from build123d import *

# Parameters (mm, degrees)
F1_DEPTH = 6.35


# Not quite as in the source:
# - a length typed as a fraction of an inch, garbled in the dataset ("3 / 203.2 mm" for 3/8 in), is restored


with BuildPart() as f1:
    # F0 (on Front) → F1 (new body)
    with BuildSketch(Plane.XZ):
        with BuildLine():
            ThreePointArc((24.579061552, 28.3529026657), (9.5195561517, 35.7531570559), (-5.2125295141, 27.720839839))
            ThreePointArc((-5.2125295141, 27.720839839), (-29.7447728029, 24.816757347), (-32.6261176355, 0.281833099))
            ThreePointArc((-32.6261176355, 0.281833099), (-47.6586884842, -25.465181848), (-20.6299769397, -38.0483339671))
            ThreePointArc((-20.6299769397, -38.0483339671), (-9.7842016961, -50.4339494071), (5.705863164, -44.8579112888))
            ThreePointArc((5.705863164, -44.8579112888), (16.7493256027, -47.8238039479), (27.779373908, -44.8084074092))
            ThreePointArc((27.779373908, -44.8084074092), (48.6340616912, -53.8941801606), (64.9161967707, -38.0082950333))
            ThreePointArc((64.9161967707, -38.0082950333), (88.8664062791, -22.618688114), (76.0994801139, 2.8265105082))
            ThreePointArc((76.0994801139, 2.8265105082), (70.0975710942, 28.7139027136), (43.5306278663, 28.0994805429))
            ThreePointArc((43.5306278663, 28.0994805429), (34.0869435906, 30.6266295541), (24.579061552, 28.3529026657))
        make_face()
        with BuildLine():
            ThreePointArc((9.9552140403, -22.4611988481), (10.8253405255, -21.564938524), (11.9872140403, -21.1061873886))
            Line((11.9872140403, -21.1061873886), (12.5920123004, -14.8077944269))
            Line((12.5920123004, -14.8077944269), (12.0265549094, -13.8484140251))
            Line((12.0265549094, -13.8484140251), (13.1350774738, -13.9548590377))
            Line((13.1350774738, -13.9548590377), (13.5390697269, -12.9171003587))
            Line((13.5390697269, -12.9171003587), (13.7382008585, -14.0127734892))
            Line((13.7382008585, -14.0127734892), (14.8467234229, -14.1192185018))
            Line((14.8467234229, -14.1192185018), (14.1090343836, -14.9534652864))
            Line((14.1090343836, -14.9534652864), (13.5042361235, -21.2518582481))
            ThreePointArc((13.5042361235, -21.2518582481), (14.3943138922, -21.7735734557), (15.0519583946, -22.5685130135))
            Line((15.0519583946, -22.5685130135), (21.1719606568, -20.9619305704))
            Line((21.1719606568, -20.9619305704), (21.788173451, -20.0343344251))
            Line((21.788173451, -20.0343344251), (22.0579849941, -21.114776255))
            Line((22.0579849941, -21.114776255), (23.1710785379, -21.1490629746))
            Line((23.1710785379, -21.1490629746), (22.2940630935, -21.8353549873))
            Line((22.2940630935, -21.8353549873), (22.5638746366, -22.9157968171))
            Line((22.5638746366, -22.9157968171), (21.5589198477, -22.4359857202))
            Line((21.5589198477, -22.4359857202), (15.4389175856, -24.0425681633))
            ThreePointArc((15.4389175856, -24.0425681633), (15.2565271687, -25.0580281222), (14.7374718125, -25.9496596209))
            Line((14.7374718125, -25.9496596209), (18.3579193376, -31.1388690552))
            Line((18.3579193376, -31.1388690552), (19.4102498473, -31.5032188374))
            Line((19.4102498473, -31.5032188374), (18.4969454746, -32.1404200522))
            Line((18.4969454746, -32.1404200522), (18.8616543221, -33.1926261736))
            Line((18.8616543221, -33.1926261736), (18.0000377843, -32.487099982))
            Line((18.0000377843, -32.487099982), (17.0867334116, -33.1243011968))
            Line((17.0867334116, -33.1243011968), (17.1080536411, -32.0108849615))
            Line((17.1080536411, -32.0108849615), (13.487606116, -26.8216755271))
            ThreePointArc((13.487606116, -26.8216755271), (12.471606116, -27.0010332485), (11.455606116, -26.8216755271))
            Line((11.455606116, -26.8216755271), (7.835158591, -32.0108849615))
            Line((7.835158591, -32.0108849615), (7.8564698266, -33.124301369))
            Line((7.8564698266, -33.124301369), (6.9431654539, -32.4871001542))
            Line((6.9431654539, -32.4871001542), (6.0815366025, -33.1926113076))
            Line((6.0815366025, -33.1926113076), (6.4462638144, -32.1404115518))
            Line((6.4462638144, -32.1404115518), (5.5329594417, -31.5032103369))
            Line((5.5329594417, -31.5032103369), (6.5852928945, -31.1388690552))
            Line((6.5852928945, -31.1388690552), (10.2057404195, -25.9496596209))
            ThreePointArc((10.2057404195, -25.9496596209), (9.6657394654, -24.9991764128), (9.5065515642, -23.9176596209))
            Line((9.5065515642, -23.9176596209), (3.4595978764, -22.0548966372))
            Line((3.4595978764, -22.0548966372), (2.4058730089, -22.4152268431))
            Line((2.4058730089, -22.4152268431), (2.7337236859, -21.3509487369))
            Line((2.7337236859, -21.3509487369), (1.7987755438, -20.7459314434))
            Line((1.7987755438, -20.7459314434), (2.9121035894, -20.7719048279))
            Line((2.9121035894, -20.7719048279), (3.2399542664, -19.7076267216))
            Line((3.2399542664, -19.7076267216), (3.9082603526, -20.5984358645))
            Line((3.9082603526, -20.5984358645), (9.9552140403, -22.4611988481))
        make_face(mode=Mode.SUBTRACT)
        with BuildLine():
            ThreePointArc((-14.9548382666, 14.9038782153), (-14.0847117815, 15.8001385395), (-12.9228382666, 16.2588896749))
            Line((-12.9228382666, 16.2588896749), (-12.3180400065, 22.5572826366))
            Line((-12.3180400065, 22.5572826366), (-12.8834973975, 23.5166630384))
            Line((-12.8834973975, 23.5166630384), (-11.7749748332, 23.4102180258))
            Line((-11.7749748332, 23.4102180258), (-11.37098258, 24.4479767047))
            Line((-11.37098258, 24.4479767047), (-11.1718514484, 23.3523035743))
            Line((-11.1718514484, 23.3523035743), (-10.0633288841, 23.2458585617))
            Line((-10.0633288841, 23.2458585617), (-10.8010179234, 22.411611777))
            Line((-10.8010179234, 22.411611777), (-11.4058161835, 16.1132188153))
            ThreePointArc((-11.4058161835, 16.1132188153), (-10.5157384147, 15.5915036078), (-9.8580939123, 14.7965640499))
            Line((-9.8580939123, 14.7965640499), (-3.7380916502, 16.4031464931))
            Line((-3.7380916502, 16.4031464931), (-3.121878856, 17.3307426383))
            Line((-3.121878856, 17.3307426383), (-2.8520673129, 16.2503008085))
            Line((-2.8520673129, 16.2503008085), (-1.7389737691, 16.2160140888))
            Line((-1.7389737691, 16.2160140888), (-2.6159892135, 15.5297220761))
            Line((-2.6159892135, 15.5297220761), (-2.3461776704, 14.4492802463))
            Line((-2.3461776704, 14.4492802463), (-3.3511324592, 14.9290913433))
            Line((-3.3511324592, 14.9290913433), (-9.4711347214, 13.3225089001))
            ThreePointArc((-9.4711347214, 13.3225089001), (-9.6535251382, 12.3070489413), (-10.1725804944, 11.4154174426))
            Line((-10.1725804944, 11.4154174426), (-6.5521329694, 6.2262080082))
            Line((-6.5521329694, 6.2262080082), (-5.4998024597, 5.8618582261))
            Line((-5.4998024597, 5.8618582261), (-6.4131068324, 5.2246570112))
            Line((-6.4131068324, 5.2246570112), (-6.0483979848, 4.1724508898))
            Line((-6.0483979848, 4.1724508898), (-6.9100145227, 4.8779770815))
            Line((-6.9100145227, 4.8779770815), (-7.8233188953, 4.2407758666))
            Line((-7.8233188953, 4.2407758666), (-7.8019986659, 5.354192102))
            Line((-7.8019986659, 5.354192102), (-11.4224461909, 10.5434015363))
            ThreePointArc((-11.4224461909, 10.5434015363), (-12.4384461909, 10.3640438149), (-13.4544461909, 10.5434015363))
            Line((-13.4544461909, 10.5434015363), (-17.0748937159, 5.354192102))
            Line((-17.0748937159, 5.354192102), (-17.0535824803, 4.2407756944))
            Line((-17.0535824803, 4.2407756944), (-17.966886853, 4.8779769093))
            Line((-17.966886853, 4.8779769093), (-18.8285157045, 4.1724657558))
            Line((-18.8285157045, 4.1724657558), (-18.4637884925, 5.2246655117))
            Line((-18.4637884925, 5.2246655117), (-19.3770928652, 5.8618667265))
            Line((-19.3770928652, 5.8618667265), (-18.3247594124, 6.2262080082))
            Line((-18.3247594124, 6.2262080082), (-14.7043118874, 11.4154174426))
            ThreePointArc((-14.7043118874, 11.4154174426), (-15.2443128415, 12.3659006506), (-15.4035007427, 13.4474174426))
            Line((-15.4035007427, 13.4474174426), (-21.4504544305, 15.3101804262))
            Line((-21.4504544305, 15.3101804262), (-22.5041792981, 14.9498502204))
            Line((-22.5041792981, 14.9498502204), (-22.176328621, 16.0141283266))
            Line((-22.176328621, 16.0141283266), (-23.1112767632, 16.61914562))
            Line((-23.1112767632, 16.61914562), (-21.9979487176, 16.5931722356))
            Line((-21.9979487176, 16.5931722356), (-21.6700980405, 17.6574503418))
            Line((-21.6700980405, 17.6574503418), (-21.0017919544, 16.7666411989))
            Line((-21.0017919544, 16.7666411989), (-14.9548382666, 14.9038782153))
        make_face(mode=Mode.SUBTRACT)
        with BuildLine():
            ThreePointArc((48.6740988512, 2.4488521783), (49.5442253363, 3.3451125024), (50.7060988512, 3.8038636378))
            Line((50.7060988512, 3.8038636378), (51.3108971112, 10.1022565995))
            Line((51.3108971112, 10.1022565995), (50.7454397202, 11.0616370013))
            Line((50.7454397202, 11.0616370013), (51.8539622846, 10.9551919887))
            Line((51.8539622846, 10.9551919887), (52.2579545378, 11.9929506677))
            Line((52.2579545378, 11.9929506677), (52.4570856693, 10.8972775372))
            Line((52.4570856693, 10.8972775372), (53.5656082337, 10.7908325246))
            Line((53.5656082337, 10.7908325246), (52.8279191944, 9.95658574))
            Line((52.8279191944, 9.95658574), (52.2231209343, 3.6581927783))
            ThreePointArc((52.2231209343, 3.6581927783), (53.113198703, 3.1364775707), (53.7708432054, 2.3415380128))
            Line((53.7708432054, 2.3415380128), (59.8908454676, 3.948120456))
            Line((59.8908454676, 3.948120456), (60.5070582618, 4.8757166012))
            Line((60.5070582618, 4.8757166012), (60.7768698049, 3.7952747714))
            Line((60.7768698049, 3.7952747714), (61.8899633487, 3.7609880518))
            Line((61.8899633487, 3.7609880518), (61.0129479043, 3.0746960391))
            Line((61.0129479043, 3.0746960391), (61.2827594474, 1.9942542093))
            Line((61.2827594474, 1.9942542093), (60.2778046585, 2.4740653062))
            Line((60.2778046585, 2.4740653062), (54.1578023964, 0.8674828631))
            ThreePointArc((54.1578023964, 0.8674828631), (53.9754119795, -0.1479770958), (53.4563566233, -1.0396085945))
            Line((53.4563566233, -1.0396085945), (57.0768041484, -6.2288180289))
            Line((57.0768041484, -6.2288180289), (58.1291346581, -6.593167811))
            Line((58.1291346581, -6.593167811), (57.2158302854, -7.2303690258))
            Line((57.2158302854, -7.2303690258), (57.5805391329, -8.2825751472))
            Line((57.5805391329, -8.2825751472), (56.7189225951, -7.5770489556))
            Line((56.7189225951, -7.5770489556), (55.8056182224, -8.2142501704))
            Line((55.8056182224, -8.2142501704), (55.8269384519, -7.1008339351))
            Line((55.8269384519, -7.1008339351), (52.2064909269, -1.9116245007))
            ThreePointArc((52.2064909269, -1.9116245007), (51.1904909269, -2.0909822221), (50.1744909269, -1.9116245007))
            Line((50.1744909269, -1.9116245007), (46.5540434018, -7.1008339351))
            Line((46.5540434018, -7.1008339351), (46.5753546374, -8.2142503426))
            Line((46.5753546374, -8.2142503426), (45.6620502647, -7.5770491278))
            Line((45.6620502647, -7.5770491278), (44.8004214133, -8.2825602812))
            Line((44.8004214133, -8.2825602812), (45.1651486252, -7.2303605254))
            Line((45.1651486252, -7.2303605254), (44.2518442526, -6.5931593106))
            Line((44.2518442526, -6.5931593106), (45.3041777053, -6.2288180289))
            Line((45.3041777053, -6.2288180289), (48.9246252304, -1.0396085945))
            ThreePointArc((48.9246252304, -1.0396085945), (48.3846242762, -0.0891253865), (48.225436375, 0.9923914055))
            Line((48.225436375, 0.9923914055), (42.1784826873, 2.8551543891))
            Line((42.1784826873, 2.8551543891), (41.1247578197, 2.4948241833))
            Line((41.1247578197, 2.4948241833), (41.4526084967, 3.5591022895))
            Line((41.4526084967, 3.5591022895), (40.5176603546, 4.164119583))
            Line((40.5176603546, 4.164119583), (41.6309884002, 4.1381461985))
            Line((41.6309884002, 4.1381461985), (41.9588390772, 5.2024243047))
            Line((41.9588390772, 5.2024243047), (42.6271451634, 4.3116151619))
            Line((42.6271451634, 4.3116151619), (48.6740988512, 2.4488521783))
        make_face(mode=Mode.SUBTRACT)
    extrude(amount=F1_DEPTH)


solid = f1.part
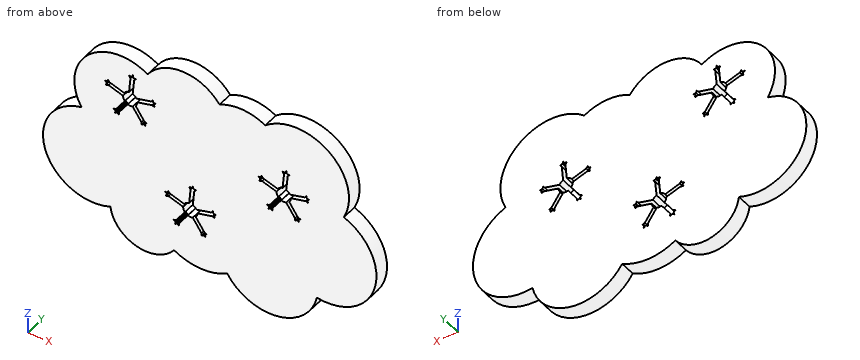
Geometry check sheet. Reference: the model listing, model coordinates, mm. Coordinates: 2 decimals unless noted, no trailing zeros. Order: outer loops, then holes, each group sorted by start corner. A loop starts at its lowest first (then second) coordinate and runs counter-clockwise, first axis right, second up. Notation, with made-up numbers: M 58.5,8.25 L 88.5,8.25 A28 ccw 88.5,27.25 Z; hole C 55,84.5 d1. An arc over 180 degrees is marked long. Use CSV: the item, a comma, the result in double quotes.
Item 1: Cross-section at A-A on z = 20. Record the cut outline in (x, y), then the cut area to 3 significant figures.
Returned:
outline,"M -33.29,-6.35 L -12.56,-6.35 L -12.56,0 L -33.29,0 Z; M -11.03,-6.35 L 76.7,-6.35 L 76.7,0 L -11.03,0 Z"
area,"689 mm2"
Item 2: Cross-section at C-C on x = 35. Record the cut outline in (y, z).
Returned:
outline,"M -6.35,-51.63 L 0,-51.63 L 0,30.59 L -6.35,30.59 Z"
Item 3: Thickness scan on line 1 along X through (y, z) = (-4, -29.5); line 2 along X through (y, z) = (-3.75, -29); line 3 along Z through (x, y) = (53, -3.5). Record the ranges inside material, lowest first.
Returned:
line 1,"x = -45.89 to 7.73, 9.59 to 15.36, 17.21 to 85.56"
line 2,"x = -46.17 to 8.08, 9.94 to 15.01, 16.87 to 85.92"
line 3,"z = -52.58 to -3.05, 3.23 to 10.15, 10.85 to 32.71"
Item 4: Cross-section at D-D on x = 69. Record the cut outline in (y, z), then the cut area to 3 significant figures.
Returned:
outline,"M -6.35,-38.27 L 0,-38.27 L 0,29.51 L -6.35,29.51 Z"
area,"430 mm2"
Item 5: Gauge pin test, flat end, axial feed: pin 1 Ø3 at (y, z) = (-4.5, -42) entering from +X. Record the tip position at first contact, or that the pin passes through.
Returned:
pin 1,"stops at x = 64.23"
Item 6: Cross-section at B-B on y = -3.5. Give the number of separate pieces and of enclosed holes in the cut face, then the cut area to 3 significant figures.
Returned:
separate pieces,"1"
enclosed holes,"3"
area,"9,090 mm2"
